Could you check a few things on this model? Use its own coordinates, in mm. A direction names the side the tool comes from. Round coordinates to 2 decimals unless told otherwise and drop trailing zeros. Write each loop counter-clockwise with the first axis right and the second up, starting at its lowest first coordinate (ties: lowest second). Pieces come first, ordered by that corner, then holes. Notation, with made-up numbers: (24, 16.25) -> (36, 16.25) arc R28 cw to (36, 54.25) -> close; hole circle Ø5 at (65.25, 88.25). An arc over 180 degrees is marked (long way). Answer in a Markdown table with one row per item.
from build123d import *

# Parameters (mm, degrees)
SKETCH1_W           = 75
SKETCH1_H           = 10
BOSS_EXTRUDE1_DEPTH = 4
SKETCH7_R           = 12.5
BOSS_EXTRUDE2_DEPTH = 4
SKETCH4_R           = 8.1
CUT_EXTRUDE3_DEPTH  = 40.730341051
FILLET2_R           = 10
SKETCH8_R           = 1.5
CUT_EXTRUDE4_DEPTH  = 40.730341051
FILLET3_R           = 5
CHAMFER1_SIZE       = 0.5


with BuildPart() as part:
    # Sketch1 → Boss-Extrude1 (new body)
    with BuildSketch(Plane(origin=(0, 0, 0), x_dir=(1, 0, 0), z_dir=(0, 1, 0))):
        Rectangle(SKETCH1_W, SKETCH1_H)
    extrude(amount=BOSS_EXTRUDE1_DEPTH)

    # Sketch7 → Boss-Extrude2 (add)
    with BuildSketch(Plane(origin=(0, 4, 0), x_dir=(1, 0, 0), z_dir=(0, 1, 0))):
        Circle(SKETCH7_R)
    extrude(amount=-BOSS_EXTRUDE2_DEPTH)

    # Sketch4 → Cut-Extrude3 (cut, through all)
    with BuildSketch(Plane(origin=(0, 4, 0), x_dir=(1, 0, 0), z_dir=(0, 1, 0))):
        with Locations(Location((0, 0, 0), (0, 0, 270))):
            Circle(SKETCH4_R)
    extrude(amount=-CUT_EXTRUDE3_DEPTH, mode=Mode.SUBTRACT)

    # Fillet2
    fillet2_edges = [part.edges().sort_by_distance(p)[0] for p in [
        (11.456439237, 2, -5),
        (11.456439237, 2, 5),
        (-11.456439237, 2, -5),
        (-11.456439237, 2, 5),
    ]]
    fillet(fillet2_edges, radius=FILLET2_R)

    # Sketch8 → Cut-Extrude4 (cut, through all)
    with BuildSketch(Plane(origin=(0, 4, 0), x_dir=(1, 0, 0), z_dir=(0, 1, 0))):
        with Locations(Location((-32, 0, 0), (0, 0, 270))):
            Circle(SKETCH8_R)
    cut_extrude4 = extrude(amount=-CUT_EXTRUDE4_DEPTH, mode=Mode.SUBTRACT)

    # Mirror2: Cut-Extrude4 across plane
    add(cut_extrude4.mirror(Plane(origin=(0, 0, 0), x_dir=(0, 0, 1), z_dir=(1, 0, 0))), mode=Mode.SUBTRACT)

    # Fillet3
    fillet3_edges = [part.edges().sort_by_distance(p)[0] for p in [
        (-37.5, 2, -5),
        (-37.5, 2, 5),
        (37.5, 2, 5),
        (37.5, 2, -5),
    ]]
    fillet(fillet3_edges, radius=FILLET3_R - 0.0001)  # a hair under: the kernel refuses the full size

    # Chamfer1
    chamfer1_edges = [part.edges().sort_by_distance(p)[0] for p in [
        (0, 0, -8.1),
        (0, 4, -8.1),
    ]]
    chamfer(chamfer1_edges, length=CHAMFER1_SIZE)


solid = part.part
1) Imagine slicing it at A-A, the plane x = 0. Please give me the cut outline in (y, z), plus the area to 3 significant figures.
Findings:
| item | result |
|---|---|
| outline | (0, -12.5) -> (4, -12.5) -> (4, -8.6) -> (3.5, -8.1) -> (0.5, -8.1) -> (0, -8.6) -> close; (0, 8.6) -> (0.5, 8.1) -> (3.5, 8.1) -> (4, 8.6) -> (4, 12.5) -> (0, 12.5) -> close |
| area | 34.7 mm^2 |
2) Imagine slicing it at B-B, the plane y = 2.9. Count the separate pieces of the cut face and the enclosed holes in it, plus the area to 3 significant figures.
Findings:
| item | result |
|---|---|
| separate pieces | 1 |
| enclosed holes | 3 |
| area | 771 mm^2 |
3) Please list where these lines run through material, in increasing order: line 1 (X direction, y = 1.35, z = 0); line 2 (X direction, y = 2.1, z = 2); line 3 (X direction, y = 1.05, z = 3.25).
Findings:
| item | result |
|---|---|
| line 1 | x = -37.5 to -33.5, -30.5 to -8.1, 8.1 to 30.5, 33.5 to 37.5 |
| line 2 | x = -37.08 to -7.85, 7.85 to 37.08 |
| line 3 | x = -36.3 to -7.42, 7.42 to 36.3 |
4) Thinking about a two-plate mould opening in Z: for faces 1 (the face through (36.07, 2.03, -3.5)), 2 (the face through (30.735, 2.028, 0.806)), 3 (the face through (-7.186, 2.021, 3.738)), 4 (the face through (-9, 0, 0)), which applies, +Z half, -Z half, draft (parallel to the pull), parting line (faces both ways), or undercut?
Findings:
| item | result |
|---|---|
| face 1 | -Z half |
| face 2 | undercut |
| face 3 | undercut |
| face 4 | draft |
5) Imagine slicing it at C-C, the plane z = -10.5. Please give me the cut outline in (x, y).
Findings:
| item | result |
|---|---|
| outline | (-6.78, 0) -> (6.78, 0) -> (6.78, 4) -> (-6.78, 4) -> close |
6) For pin 1 (1.2 mm diameter, centred on x = -21, y = 1.5, fed in from +Z); pin 2 (1.2 mm diameter, centred on x = -27.5, y = 2.5, fed in from -Z); pin 3 (5 mm diameter, centred on x = -16.5, z = -9.5, fed in from -Y) (1 decimal), each with a flat end and sliding along its axis, tell me the tip position at first contact or that it passes through.
Findings:
| item | result |
|---|---|
| pin 1 | stops at z = 5 |
| pin 2 | stops at z = -5 |
| pin 3 | passes through |
7) For faces 5 (the face through (-25, 2, -5)), 6 (the face through (0.1, 2, -12.5)), 7 (the face through (25, 2, -5)), 8 (the face through (-25, 2, 5)), 9 (the face through (25, 2, 5)), which set-ups out of +Z, -Z, +X, -X, +Y, -Y let a thin tool reach every point of the face, with its end or its side?
Findings:
| item | result |
|---|---|
| face 5 | -Z, -X, +Y, -Y |
| face 6 | -Z, +Y, -Y |
| face 7 | -Z, +X, +Y, -Y |
| face 8 | +Z, -X, +Y, -Y |
| face 9 | +Z, +X, +Y, -Y |
8) Imagine slicing it at D-D, the plane x = 12. Please give me the cut outline in (y, z).
Findings:
| item | result |
|---|---|
| outline | (0, -6.21) -> (4, -6.21) -> (4, 6.21) -> (0, 6.21) -> close |
